from build123d import *

# Parameters (mm, degrees)
BOSS_EXTRUDE1_DEPTH  = 6
FILLET1_R            = 10
SKETCH2_OUTSIDE_W    = 330.112
SKETCH2_OUTSIDE_H    = 380.112
SKETCH2_OUTSIDE_W_2  = 6
SKETCH2_OUTSIDE_H_2  = 49
CUT_EXTRUDE1_DEPTH   = 7
CUT_EXTRUDE2_DEPTH   = 7
LPATTERN1_COUNT      = 2
LPATTERN1_PITCH      = 245
LPATTERN1_COUNT_DIR2 = 2
LPATTERN1_PITCH_DIR2 = 210


with BuildPart() as part:
    # Sketch1 → Boss-Extrude1 (new body)
    with BuildSketch(Plane(origin=(0, 0, 0), x_dir=(1, 0, 0), z_dir=(0, 1, 0))):
        Polygon((-164.115526796, 87.380429132), (-124.115526796, 87.380429132), (-124.115526796, -112.619570868), (45.884473204, -112.619570868), (45.884473204, 87.380429132), (85.884473204, 87.380429132), (85.884473204, -212.619570868), (-164.115526796, -212.619570868), align=None)
    extrude(amount=BOSS_EXTRUDE1_DEPTH)

    # Fillet1
    fillet1_edges = [part.edges().sort_by_distance(p)[0] for p in [
        (-164.115526796, 3, -87.380429132),
        (-124.115526796, 3, -87.380429132),
        (-124.115526796, 3, 112.619570868),
        (45.884473204, 3, 112.619570868),
        (45.884473204, 3, -87.380429132),
        (85.884473204, 3, -87.380429132),
        (85.884473204, 3, 212.619570868),
        (-164.115526796, 3, 212.619570868),
    ]]
    fillet(fillet1_edges, radius=FILLET1_R)

    # Sketch2 outside → Cut-Extrude1 (cut, through all)
    with BuildSketch(Plane.XZ):
        with Locations((-39.116, 62.62)):
            Rectangle(SKETCH2_OUTSIDE_W, SKETCH2_OUTSIDE_H)
        with BuildLine():
            Line((-164.115526796, 202.619570868), (-164.115526796, -77.380429132))
            ThreePointArc((-164.115526796, -77.380429132), (-161.186594608, -84.451496944), (-154.115526796, -87.380429132))
            Line((-154.115526796, -87.380429132), (-134.115526796, -87.380429132))
            ThreePointArc((-134.115526796, -87.380429132), (-127.044458984, -84.451496944), (-124.115526796, -77.380429132))
            Line((-124.115526796, -77.380429132), (-124.115526796, 102.619570868))
            ThreePointArc((-124.115526796, 102.619570868), (-121.186594608, 109.69063868), (-114.115526796, 112.619570868))
            Line((-114.115526796, 112.619570868), (35.884473204, 112.619570868))
            ThreePointArc((35.884473204, 112.619570868), (42.955541016, 109.69063868), (45.884473204, 102.619570868))
            Line((45.884473204, 102.619570868), (45.884473204, -77.380429132))
            ThreePointArc((45.884473204, -77.380429132), (48.813405392, -84.451496944), (55.884473204, -87.380429132))
            Line((55.884473204, -87.380429132), (75.884473204, -87.380429132))
            ThreePointArc((75.884473204, -87.380429132), (82.955541016, -84.451496944), (85.884473204, -77.380429132))
            Line((85.884473204, -77.380429132), (85.884473204, 202.619570868))
            ThreePointArc((85.884473204, 202.619570868), (82.955541016, 209.69063868), (75.884473204, 212.619570868))
            Line((75.884473204, 212.619570868), (-154.115526796, 212.619570868))
            ThreePointArc((-154.115526796, 212.619570868), (-161.186594608, 209.69063868), (-164.115526796, 202.619570868))
        make_face(mode=Mode.SUBTRACT)
        with Locations((-52.115526796, 148.119570868)):
            Rectangle(SKETCH2_OUTSIDE_W_2, SKETCH2_OUTSIDE_H_2)
        with Locations((-26.115526796, 148.119570868)):
            Rectangle(SKETCH2_OUTSIDE_W_2, SKETCH2_OUTSIDE_H_2)
    extrude(amount=-CUT_EXTRUDE1_DEPTH, mode=Mode.SUBTRACT)

    # Sketch5 → Cut-Extrude2 (cut, through all)
    with BuildSketch(Plane(origin=(0, 0, 0), x_dir=(-1, 0, 0), z_dir=(0, -1, 0))):
        with BuildLine():
            Line((134.115526796, 58.380429132), (140.76142483, 58.380429132))
            ThreePointArc((140.76142483, 58.380429132), (144.115526796, 56.880429132), (147.469628762, 58.380429132))
            Line((147.469628762, 58.380429132), (154.115526796, 58.380429132))
            Line((154.115526796, 58.380429132), (154.115526796, 64.380429132))
            Line((154.115526796, 64.380429132), (147.469628762, 64.380429132))
            ThreePointArc((147.469628762, 64.380429132), (144.115526796, 65.880429132), (140.76142483, 64.380429132))
            Line((140.76142483, 64.380429132), (134.115526796, 64.380429132))
            Line((134.115526796, 64.380429132), (134.115526796, 58.380429132))
        make_face()
    cut_extrude2 = extrude(amount=-CUT_EXTRUDE2_DEPTH, mode=Mode.SUBTRACT)

    # LPattern1: Cut-Extrude2 2 × 2
    with Locations(*[(j * LPATTERN1_PITCH_DIR2, 0, i * LPATTERN1_PITCH) for i in range(LPATTERN1_COUNT) for j in range(LPATTERN1_COUNT_DIR2) if (i, j) != (0, 0)]):
        add(cut_extrude2, mode=Mode.SUBTRACT)


solid = part.part
Read the model definition and answer for the solid it produces. Units are mm, in the model's axes. A direction names the side the tool comes from. Round coordinates to 2 decimals unless told otherwise and drop trailing zeros. Write each loop counter-clockwise with the first axis right and the second up, starting at its lowest first coordinate (ties: lowest second). Pieces come first, ordered by that corner, then holes.
Q1. A tool of negligible diameter and unlimited length cuts with its end or side. For faces 1 (the face through (59, 3, 186.62)), 2 (the face through (42.877, 3.042, 109.768)), 3 (the face through (83.033, 3.042, 209.612)), from which of +Z, -Z, +X, -X, +Y, -Y can it reach the whole face along a straight path? Write none if from no direction.
Values:
face 1: +Y, -Y
face 2: -Z, +Y, -Y
face 3: +Z, +X, +Y, -Y
Q2. Find section C-C on y = 3.6. State how many separate pieces and enclosed holes the cut face has, and give its area (3 significant figures).
Values:
separate pieces: 1
enclosed holes: 6
area: 39,800 mm2
Q3. A flat-ended cylindrical pin translates along its axis: P1, Ø2, axis at x = -27.5, y = 4.5, coming from the -Z side. Find the tip coordinate at first contact, or state that the pin passes through.
Values:
P1: stops at z = 112.62
Q4. Straight lines are drawn through the part: line 1 (Z direction, x = -139, y = 2.45); line 2 (X direction, y = 1.55, z = 144.5); line 3 (X direction, y = 1.35, z = 95). For each, find the intervals that lie inside material, in ascending order.
Values:
line 1: z = -87.38 to -64.38, -58.38 to 180.62, 186.62 to 212.62
line 2: x = -164.12 to -55.12, -49.12 to -29.12, -23.12 to 85.88
line 3: x = -164.12 to -124.12, 45.88 to 85.88
Q5. Find section B-B on z = 158. Determine the outline of the cut face in (x, y), and give its area (3 significant figures).
Values:
outline: (-164.12, 0) - (-55.12, 0) - (-55.12, 6) - (-164.12, 6) - close; (-49.12, 0) - (-29.12, 0) - (-29.12, 6) - (-49.12, 6) - close; (-23.12, 0) - (85.88, 0) - (85.88, 6) - (-23.12, 6) - close
area: 1,430 mm2
Q6. Find section D-D on x = -65. Determine the outline of the cut face in (y, z), and give its area (3 significant figures).
Values:
outline: (0, 112.62) - (6, 112.62) - (6, 212.62) - (0, 212.62) - close
area: 600 mm2
Q7. The mould has two halves that part along Z. Classify faces 4 (the face through (65.83, 2.96, -65.88)), 5 (the face through (-151, 3, 180.62)), 6 (the face through (-161.108, 3.042, 209.768)), 7 (the face through (82.877, 3.042, -84.529)): released by +Z, released by -Z, zero draft, split by the parting line, or undercut.
Values:
face 4: undercut
face 5: undercut
face 6: released by +Z
face 7: released by -Z
Q8. Find section A-A on z = 86. Determine the outline of the cut face in (x, y), and give its area (3 significant figures).
Values:
outline: (-164.12, 0) - (-124.12, 0) - (-124.12, 6) - (-164.12, 6) - close; (45.88, 0) - (85.88, 0) - (85.88, 6) - (45.88, 6) - close
area: 480 mm2
